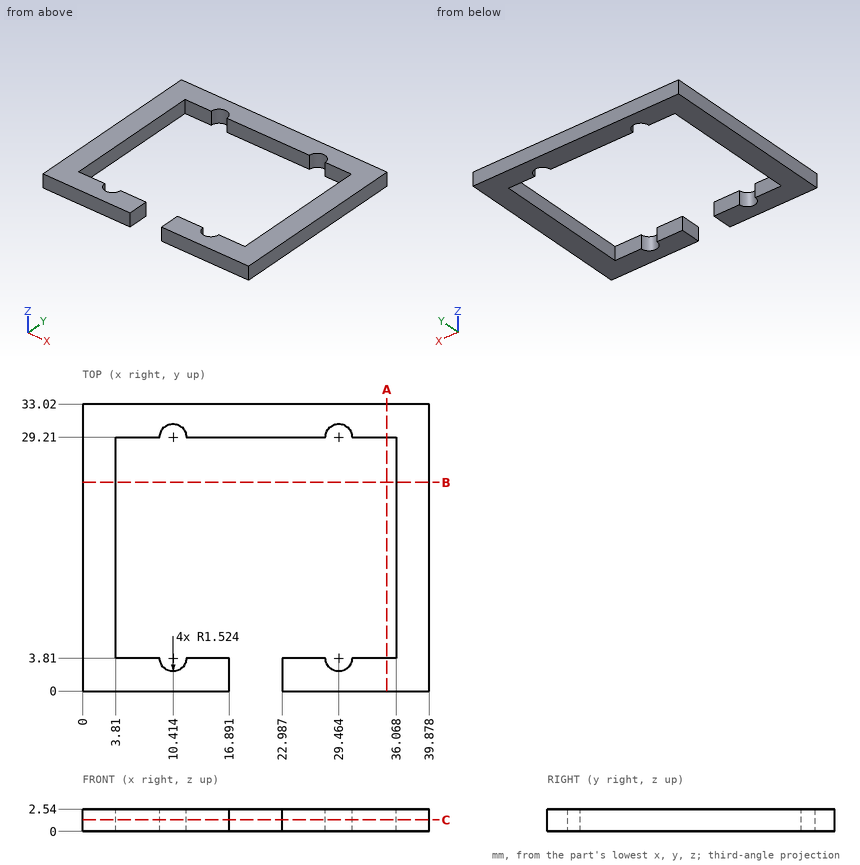
Part print with two shaded views. Sizes in mm from the minimum x, y, z corner. Coordinates: 2 decimals unless noted, no trailing zeros. Write each loop counter-clockwise with the first axis right and the second up, starting at its lowest first coordinate (ties: lowest second). Pieces come first, ordered by that corner, then holes. Notation, with made-up numbers: (8.25, 49.5) - (48.25, 49.5) arc R6 cw to (48.25, 53.5) - close; hole circle Ø2 at (-11.5, -28.75). An arc over 180 degrees is marked (long way). Use a Markdown table: item, result. Add a question column.
Item 1: Band-saw the part on B-B, the plane y = 24. Write the cut outline in (x, z), and give its area (3 significant figures).
Item 2: Drop a flat-ended pin along its axis: pin 1 (0.8 mm diameter, centred on x = 18, z = 2, fed in from -Y). Give the stop position or say it passes through.
Item 3: Drill centre lines: line 1 along Y through (x, z) = (32, 0.5); line 2 along X through (y, z) = (20, 0.8); line 3 along X through (y, z) = (2.5, 1.6). Where is each one in solid material? Low to high.
Item 4: Band-saw the part on C-C, the plane z = 1.3. Write the cut outline in (x, y).
Item 5: Band-saw the part on A-A, the plane x = 35. Write the cut outline in (y, z).
A:
| question | item | result |
|---|---|---|
| 1 | outline | (0, 0) - (3.81, 0) - (3.81, 2.54) - (0, 2.54) - close; (36.07, 0) - (39.88, 0) - (39.88, 2.54) - (36.07, 2.54) - close |
| 1 | area | 19.4 mm² |
| 2 | pin 1 | stops at y = 29.21 |
| 3 | line 1 | y = 0 to 3.81, 29.21 to 33.02 |
| 3 | line 2 | x = 0 to 3.81, 36.07 to 39.88 |
| 3 | line 3 | x = 0 to 9.64, 11.19 to 16.89, 22.99 to 28.69, 30.24 to 39.88 |
| 4 | outline | (0, 0) - (16.89, 0) - (16.89, 3.81) - (11.94, 3.81) arc R1.52 cw to (8.89, 3.81) - (3.81, 3.81) - (3.81, 29.21) - (8.89, 29.21) arc R1.52 cw to (11.94, 29.21) - (27.94, 29.21) arc R1.52 cw to (30.99, 29.21) - (36.07, 29.21) - (36.07, 3.81) - (30.99, 3.81) arc R1.52 cw to (27.94, 3.81) - (22.99, 3.81) - (22.99, 0) - (39.88, 0) - (39.88, 33.02) - (0, 33.02) - close |
| 5 | outline | (0, 0) - (3.81, 0) - (3.81, 2.54) - (0, 2.54) - close; (29.21, 0) - (33.02, 0) - (33.02, 2.54) - (29.21, 2.54) - close |
